Verification items for this drawing (mm, ordinates from the low corner). Round coordinates to 2 decimals unless told otherwise and drop trailing zeros. Order: outer loops, then holes, each group sorted by start corner. A loop starts at its lowest first (then second) coordinate and runs counter-clockwise, first axis right, second up. Notation, with made-up numbers: M 72.5,18.25 L 87.5,18.25 A30 cw 87.5,55.25 Z; hole C 22,-19.75 d3. An arc over 180 degrees is marked long. Use CSV: the item, a comma, the result in double quotes. Start each with the question number.
Q1. Sectioned sample at B-B (z = 0.75). State how many separate pieces and enclosed holes the cut face has.
Q2. Scan lines: line 1 (X direction, y = 17, z = 2) (1 decimal); line 2 (Y direction, x = 27, z = 0.65) (1 decimal); line 3 (Y direction, x = 132.5, z = 2.3). Record each from-to range of solid material in increasing order.
Q3. Sectioned sample at C-C (y = 24). Enter the section's corners in (x, z).
Q4. Sectioned sample at A-A (y = 6). Enter the section's corners in (x, z).
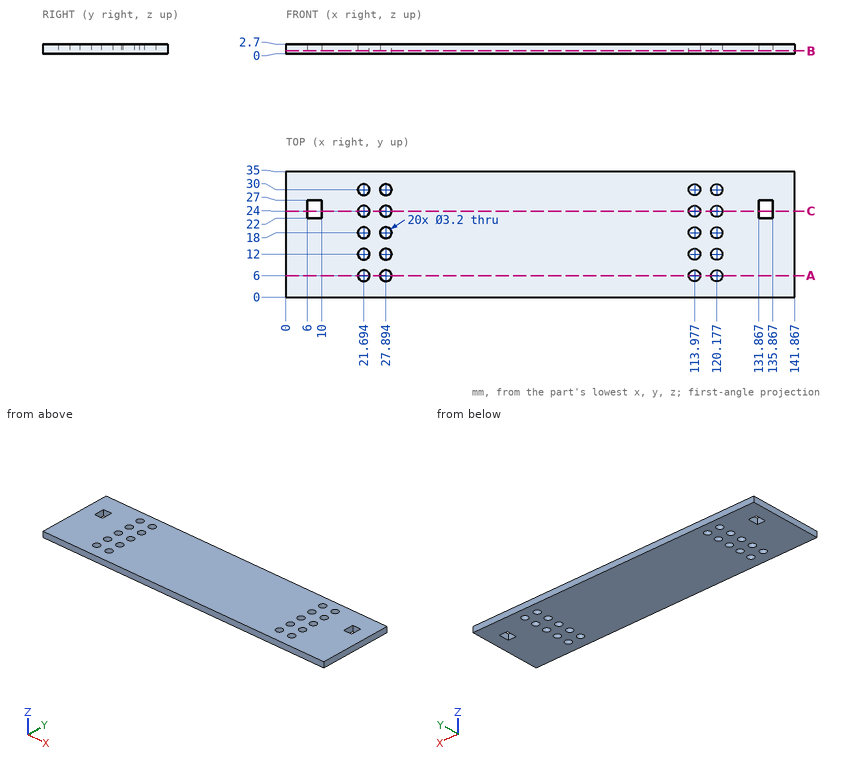
Verdict:
1,separate pieces,"1"
1,enclosed holes,"22"
2,line 1,"x = 0 to 20.4, 22.9 to 26.6, 29.1 to 112.7, 115.2 to 118.9, 121.4 to 141.9"
2,line 2,"y = 0 to 4.7, 7.3 to 10.7, 13.3 to 16.7, 19.3 to 22.7, 25.3 to 28.7, 31.3 to 35"
2,line 3,"y = 0 to 22, 27 to 35"
3,outline,"M 0,0 L 6,0 L 6,2.7 L 0,2.7 Z; M 10,0 L 20.09,0 L 20.09,2.7 L 10,2.7 Z; M 23.29,0 L 26.29,0 L 26.29,2.7 L 23.29,2.7 Z; M 29.49,0 L 112.38,0 L 112.38,2.7 L 29.49,2.7 Z; M 115.58,0 L 118.58,0 L 118.58,2.7 L 115.58,2.7 Z; M 121.78,0 L 131.87,0 L 131.87,2.7 L 121.78,2.7 Z; M 135.87,0 L 141.87,0 L 141.87,2.7 L 135.87,2.7 Z"
4,outline,"M 0,0 L 20.09,0 L 20.09,2.7 L 0,2.7 Z; M 23.29,0 L 26.29,0 L 26.29,2.7 L 23.29,2.7 Z; M 29.49,0 L 112.38,0 L 112.38,2.7 L 29.49,2.7 Z; M 115.58,0 L 118.58,0 L 118.58,2.7 L 115.58,2.7 Z; M 121.78,0 L 141.87,0 L 141.87,2.7 L 121.78,2.7 Z"
